CAD build for the part. Positions are in the model's coordinates, mm. Face numbers are marked on the shaded views. A direction names the side the tool comes from. Coordinates: 2 decimals unless noted, no trailing zeros. Order: outer loops, then holes, each group sorted by start corner. A loop starts at its lowest first (then second) coordinate and runs counter-clockwise, first axis right, second up. Notation, with made-up numbers: (53.5, 76.5) - (62.5, 76.5) arc R24 cw to (62.5, 89.5) - close; hole circle Ø3 at (-26.75, 79.25). An arc over 180 degrees is marked (long way). Write each question's results on one line, items separated by ' | '. Start each with the question number.
Q1. Band-saw the part on B-B, the plane y = 10.5. Write the cut outline in (x, z).
Q2. Band-saw the part on C-C, the plane x = -9. Write the cut outline in (y, z), then the cut area to 3 significant figures.
Q3. Pull direction X, two halves, no side cores. Call the marked faces 1, 2 and 3: released by +X, released by -X, zero draft, split by the parting line, or undercut.
Q4. Which spindle directions (+Z, -Z, +X, -X, +Y, -Y) get a long thin tool onto all of the face, cutting with end or side? Do the marked faces 4 and 5. Say none if no direction does.
Q5. Wall check: probe 1 along X at (y, z) = (2, 0); probe 2 along X at (y, z) = (1.7, 0); probe 3 along X at (y, z) = (4.75, 2.25). Give the ranges that are in metal, low to high.
Q6. Band-saw the part on D-D, the plane z = -6.25. Write the cut outline in (x, y).
Q7. Band-saw the part on A-A, the plane z = 0. Count the separate pieces of the cut face and the enclosed holes in it, then the cut area to 3 significant figures.
Autodesk Inventor part; units mm, degrees
ref_plane "YZ Plane" through (0, 0, 0) normal (1, 0, 0) x (0, 1, 0)
ref_plane "XZ Plane" through (0, 0, 0) normal (0, 1, 0) x (-1, 0, 0)
ref_plane "XY Plane" through (0, 0, 0) normal (0, 0, 1) x (1, 0, 0)
sketch "Эскиз1" plane through (0, 0, 0) normal (0, 1, 0) x (-1, 0, 0)
  line L0 (11.5, -8) -> (-11.5, -8)
  line L1 (-11.5, -8) -> (-11.5, 8)
  line L2 (-11.5, 8) -> (11.5, 8)
  line L3 (11.5, 8) -> (11.5, -8)
  line L4 (11.5, -8) -> (-11.5, 8) construction
  line L5 (-11.5, -8) -> (11.5, 8) construction
  point P0 (0, 0)
  dimension "d0" = 23
  dimension "d1" = 16
extrude "Выдавливание1" add sketch "Эскиз1" along normal blind 11.5
sketch "Эскиз2" plane through (-11.5, 0, 8) normal (0, 0, 1) x (1, 0, 0)
  line L0 (0, 0) -> (0, 11.5)
  line L1 (23, 0) -> (8.5, 0) construction
  line L2 (8.5, 0) -> (8.5, 4) construction
  line L3 (8.5, 4) -> (23, 4) construction
  line L4 (23, 4) -> (23, 0) construction
  line L5 (23, 0) -> (21, 0) construction
  line L6 (21, 0) -> (21, 5.75) construction
  line L7 (21, 5.75) -> (23, 5.75) construction
  line L8 (23, 5.75) -> (23, 0) construction
  circle A0 centre (8.5, 4) radius 3
  circle A1 centre (21, 5.75) radius 1.55
  line L9 (-8.5, 3.5) -> (8.5, 3.5)
  line L10 (8.5, 3.5) -> (8.5, 4.5)
  line L11 (8.5, 4.5) -> (-8.5, 4.5)
  line L12 (-8.5, 4.5) -> (-8.5, 3.5)
  line L13 (-8.5, 3.5) -> (8.5, 4.5) construction
  line L14 (8.5, 3.5) -> (-8.5, 4.5) construction
  point P0 (11.5, 0)
  point P1 (0, 4)
  dimension "d4" = 14.5
  dimension "d5" = 4
  dimension "d6" = 2
  dimension "d7" = 5.75
  dimension "d8" = 6
  dimension "d9" = 3.1
  dimension "d10" = 1
extrude "Выдавливание2" cut sketch "Эскиз2" against normal up to next
sketch "Эскиз3" plane through (0, 11.5, 0) normal (0, 1, 0) x (1, 0, 0)
  line L0 (11.5, -8) -> (11.5, 8)
  line L1 (11.5, 0) -> (-9, 0) construction
  line L2 (11.5, 0) -> (3.5, 0) construction
  circle A0 centre (-9, 0) radius 1.5
  circle A1 centre (3.5, 0) radius 3
  point P0 (0, 0)
  dimension "d13" = 20.5
  dimension "d14" = 8
  dimension "d15" = 3
  dimension "d16" = 6
extrude "Выдавливание3" cut sketch "Эскиз3" against normal up to surface (11.5 mm away)
sketch "Эскиз4" plane through (0, 0, 0) normal (0, -1, 0) x (1, 0, 0)
  line L0 (11.5, -8) -> (11.5, 8)
  line L1 (-11.5, 8) -> (-11.5, -8)
  line L2 (11.5, 0) -> (9.5, 0) construction
  circle A0 centre (9.5, 0) radius 1.5
  point P0 (0, 0)
  dimension "d19" = 2
  dimension "d20" = 3
extrude "Выдавливание4" cut sketch "Эскиз4" against normal up to next
fillet "Сопряжение1" radius 0.5 14 edges at (0, 11.5, 8) (11.5, 11.5, 0) (11.5, 5.75, 8) (11.5, 0, 0) (11.5, 5.75, -8) (0, 11.5, -8) (-11.5, 11.5, 0) (0, 0, 8) (-11.5, 0, 0) (0, 0, -8) (-11.5, 1.75, 8) (-11.5, 8, 8) (-11.5, 8, -8) (-11.5, 1.75, -8)
thread "Резьба1"
thread "Резьба2"
thread "Резьба3"
thread "Резьба4"
properties part number "BLOCK-CARTRIDGE"
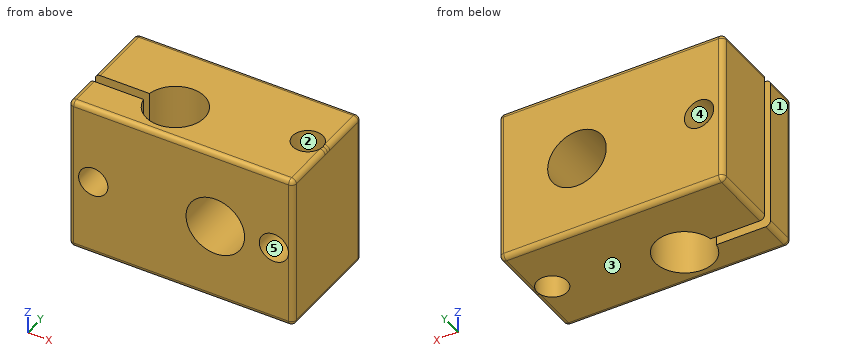
Results below:
1) outline: (-11.5, -7.5) arc R0.5 ccw to (-11, -8) - (11, -8) arc R0.5 ccw to (11.5, -7.5) - (11.5, 7.5) arc R0.5 ccw to (11, 8) - (-11, 8) arc R0.5 ccw to (-11.5, 7.5) - close; hole circle Ø3 at (-9, 0); hole circle Ø6 at (3.5, 0)
2) outline: (0, -7.5) arc R0.5 ccw to (0.5, -8) - (3.5, -8) - (3.5, -1.5) - (0, -1.5) - close; (0, 1.5) - (3.5, 1.5) - (3.5, 8) - (0.5, 8) arc R0.5 ccw to (0, 7.5) - close; (4.5, -8) - (11, -8) arc R0.5 ccw to (11.5, -7.5) - (11.5, -1.5) - (4.5, -1.5) - close; (4.5, 1.5) - (11.5, 1.5) - (11.5, 7.5) arc R0.5 ccw to (11, 8) - (4.5, 8) - close | area: 136 mm²
3) face 1: released by -X | face 2: undercut | face 3: zero draft
4) face 4: +Y, -Y | face 5: -Y
5) probe 1: x = -11.5 to -10.5, -7.5 to -5.24, -0.76 to 0.5, 6.5 to 8, 11 to 11.5 | probe 2: x = -11.5 to -10.5, -7.5 to -4.93, -1.07 to 0.5, 6.5 to 8, 11 to 11.5 | probe 3: x = -11.5 to -5.9, -0.1 to 1.52, 5.48 to 8.32, 10.68 to 11.5
6) outline: (-11.5, 0.5) arc R0.5 ccw to (-11, 0) - (11, 0) arc R0.5 ccw to (11.5, 0.5) - (11.5, 11) arc R0.5 ccw to (11, 11.5) - (-11, 11.5) arc R0.5 ccw to (-11.5, 11) - (-11.5, 4.5) - (-5.96, 4.5) arc R3 cw (long way) to (-5.96, 3.5) - (-11.5, 3.5) - close; hole circle Ø3.1 at (9.5, 5.75)
7) separate pieces: 4 | enclosed holes: 0 | area: 109 mm²
